```python
from build123d import *

# Parameters (mm, degrees)
SKETCH_1_W          = 87
SKETCH_1_H          = 58
SKETCH_1_W_2        = 4
SKETCH_1_H_2        = 18
EXTRUDE_1_DEPTH     = 2
SKETCH_2_W          = 2
SKETCH_2_H          = 58
EXTRUDE_2_DEPTH     = 33
SKETCH_3_R          = 1.6
EXTRUDE_3_DEPTH     = 2
CUT_EXTRUDE_1_REACH = 69.203
SKETCH_4_W          = 46.038149354
SKETCH_4_H          = 33.396976304


with BuildPart() as part:
    # 草图1 → 凸台-拉伸1 (new body)
    with BuildSketch(Plane(origin=(0, 0, 0), x_dir=(1, 0, 0), z_dir=(0, 1, 0))):
        Rectangle(SKETCH_1_W, SKETCH_1_H)
        with Locations((45.5, 4)):
            Rectangle(SKETCH_1_W_2, SKETCH_1_H_2)
    extrude(amount=EXTRUDE_1_DEPTH)

    # 草图2 → 凸台-拉伸2 (add)
    with BuildSketch(Plane.XZ):
        with Locations((-42.5, 0)):
            Rectangle(SKETCH_2_W, SKETCH_2_H)
    extrude(amount=EXTRUDE_2_DEPTH)

    # 草图3 → 凸台-拉伸3 (add)
    # profile 1 of 3: a face of its own
    with BuildSketch(Plane.XZ.offset(33)):
        with BuildLine():
            Line((-43.5, 23), (-43.5, 29))
            Line((-43.5, 29), (-47.5, 29))
            ThreePointArc((-47.5, 29), (-48.914213562, 28.414213562), (-49.5, 27))
            Line((-49.5, 27), (-49.5, 25))
            ThreePointArc((-49.5, 25), (-48.914213562, 23.585786438), (-47.5, 23))
            Line((-47.5, 23), (-43.5, 23))
        make_face()
        with Locations(Location((-46.5, 26, 0), (0, 0, 270))):
            Circle(SKETCH_3_R, mode=Mode.SUBTRACT)
    # profile 2 of 3: a face of its own
    with BuildSketch(Plane.XZ.offset(33)):
        Polygon((-41.5, 29), (-43.5, 29), (-43.5, 23), (-43.5, -23), (-43.5, -29), (-41.5, -29), align=None)
    # profile 3 of 3: a face of its own
    with BuildSketch(Plane.XZ.offset(33)):
        with BuildLine():
            Line((-43.5, -29), (-43.5, -23))
            Line((-43.5, -23), (-47.5, -23))
            ThreePointArc((-47.5, -23), (-48.914213562, -23.585786438), (-49.5, -25))
            Line((-49.5, -25), (-49.5, -27))
            ThreePointArc((-49.5, -27), (-48.914213562, -28.414213562), (-47.5, -29))
            Line((-47.5, -29), (-43.5, -29))
        make_face()
        with Locations(Location((-46.5, -26, 0), (0, 0, 270))):
            Circle(SKETCH_3_R, mode=Mode.SUBTRACT)
    extrude(amount=-EXTRUDE_3_DEPTH)

    # 草图4 → 切除-拉伸1 (cut, up to next)
    with BuildSketch(Plane(origin=(0, 2, 0), x_dir=(1, 0, 0), z_dir=(0, 1, 0)), mode=Mode.PRIVATE) as cut_extrude_1_sk1:
        with Locations((-0.850083312, -0.605075521)):
            Rectangle(SKETCH_4_W, SKETCH_4_H)
    cut_extrude_1_tool1 = extrude(cut_extrude_1_sk1.sketch, amount=-CUT_EXTRUDE_1_REACH, mode=Mode.PRIVATE) & part.part
    add(cut_extrude_1_tool1.solids().sort_by_distance((-0.850083, 2, 0.605076))[0], mode=Mode.SUBTRACT)


solid = part.part
```
Can you work these out from the model? Positions are in its coordinate system, mm. A direction names the side the tool comes from. Give positions to 0.01 mm unless a question says otherwise; leave off trailing zeros. Loops run counter-clockwise (first coordinate to the right, second up) from the corner with the lowest first, then second, coordinate; pieces in that order, holes last. Notation, with made-up numbers: M 47.5,31 L 68.5,31 A8 cw 68.5,42 Z; hole C 88.5,59.25 d6. An arc over 180 degrees is marked long. Use one line per item in the form item = value. Start each with the question number.
(1) Thinking about a two-plate mould opening in Z: for faces 1 (the flat face through (-22, 1, 29)), 2 (the flat face through (-45, -31, 25)), 3 (the cylindrical face through (-48.93, -32.01, 23.6)), which applies, released by +Z, released by -Z, zero draft, split by the parting line, or undercut?
(2) I want a section at B-B, the plane x = 9. Write out the boundary of the cut face in (y, z), and give its area (3 significant figures).
(3) Please list where these lines run through material, in increasing order: line 1 (X direction, y = -32.1, z = -26); line 2 (X direction, y = -22, z = 10); line 3 (Z direction, x = -46, y = -32).
(4) I want a section at D-D, the plane z = 9.5. Write out the boundary of the cut face in (x, y), and give its area (3 significant figures).
(5) I want a section at A-A, the plane z = 3. Write out the boundary of the cut face in (x, y).
(6) I'm going to push flat-ended pins straight in: P1, Ø5, axis at y = -18.5, z = -1.5, coming from the +X side; P2, Ø1.6, axis at y = 0.5, z = -18.5, coming from the +X side; P3, Ø1, axis at x = 45.5, y = 1, coming from the -Z side. Where does each tip first touch, or does it pass through?
(7) I want a section at C-C, the plane x = -46.5. Write out the boundary of the cut face in (y, z).
(8) On a 3-axis mill with a long thin cutter (end or side, diameter ignored), from which of +Z, -Z, +X, -X, +Y, -Y can I reach the whole of each face in a straight line? I mean faces 4 (the flat face through (-41.5, -16, 0)), 5 (the flat face through (-45, -31, -27)), 6 (the cylindrical face through (-48.9, -32.01, -23.57)), 7 (the flat face through (43.5, 1, 17)), 8 (the flat face through (-23.869, 1, 1)). Say none if no direction works.
Worked out:
q1.face_1 = released by +Z
q1.face_2 = zero draft
q1.face_3 = undercut
q2.outline = M 0,-29 L 2,-29 L 2,-16.09 L 0,-16.09 Z; M 0,17.3 L 2,17.3 L 2,29 L 0,29 Z
q2.area = 49.2 mm²
q3.line_1 = -49.5 to -48.1, -44.9 to -41.5
q3.line_2 = -43.5 to -41.5
q3.line_3 = -29 to -27.52, -24.48 to -23, 23 to 24.48, 27.52 to 29
q4.outline = M -43.5,-33 L -41.5,-33 L -41.5,0 L -23.87,0 L -23.87,2 L -43.5,2 Z; M 22.17,0 L 43.5,0 L 43.5,2 L 22.17,2 Z
q4.area = 148 mm²
q5.outline = M -43.5,-33 L -41.5,-33 L -41.5,0 L -23.87,0 L -23.87,2 L -43.5,2 Z; M 22.17,0 L 47.5,0 L 47.5,2 L 22.17,2 Z
q6.P1 = -41.5
q6.P2 = 43.5
q6.P3 = -13
q7.outline = M -33,-29 L -31,-29 L -31,-27.6 L -33,-27.6 Z; M -33,-24.4 L -31,-24.4 L -31,-23 L -33,-23 Z; M -33,23 L -31,23 L -31,24.4 L -33,24.4 Z; M -33,27.6 L -31,27.6 L -31,29 L -33,29 Z
q8.face_4 = +Z, -Z, +X, -Y
q8.face_5 = +Z, -Z, -X, +Y
q8.face_6 = -X, +Y, -Y
q8.face_7 = +Z, +X, +Y, -Y
q8.face_8 = +Y, -Y
